Can you work these out from the model? Positions are in its coordinate system, mm. Face numbers are marked on the shaded views. A direction names the side the tool comes from. Give positions to 0.01 mm unless a question says otherwise; leave off trailing zeros. Loops run counter-clockwise (first coordinate to the right, second up) from the corner with the lowest first, then second, coordinate; pieces in that order, holes last. Notation, with made-up numbers: M -11.5,67 L -5.5,67 A23 ccw -5.5,90 Z; hole C 86,-6 d10. An arc over 180 degrees is marked long. Put each result on its own line as item: value. Start each with the question number.
1) Imagine slicing it at D-D (x = 5.5). Write out the boundary of the cut face in (y, z).
2) Imagine slicing it at B-B (z = 3.3). Write out the boundary of the cut face in (x, y).
3) For P1, Ø1.8, axis at x = 16.35, y = 10, coming from the -Z side; P2, Ø2, axis at x = 6, z = 0.5, coming from the -Y side; P3, Ø2, axis at y = 12, z = 1.5, coming from the -X side, each with a flat end and sliding along its axis, tell me the tip position at first contact or that it passes through.
4) Please list where these lines run through material, in increasing order: line 1 along Y through (x, z) = (26.35, 2.7); line 2 along X through (y, z) = (3, 0.8); line 3 along Y through (x, z) = (5, 3.45). Write a range as from..to.
5) Imagine slicing it at A-A (x = 26.35). Write out the boundary of the cut face in (y, z).
6) Imagine slicing it at C-C (y = 2.5). Write out the boundary of the cut face in (x, z), then the cut area to 3 significant figures.
7) For the marked faces 1, 2 and 3, which set-ups out of +Z, -Z, +X, -X, +Y, -Y let a thin tool reach every point of the face, with its end or its side?
8) If we mould it in two halves opening along Y, with no side actions, what happens to the marked faces 4, 5 and 6? For each: +Y half, -Y half, draft (parallel to the pull), parting line (faces both ways), or undercut.
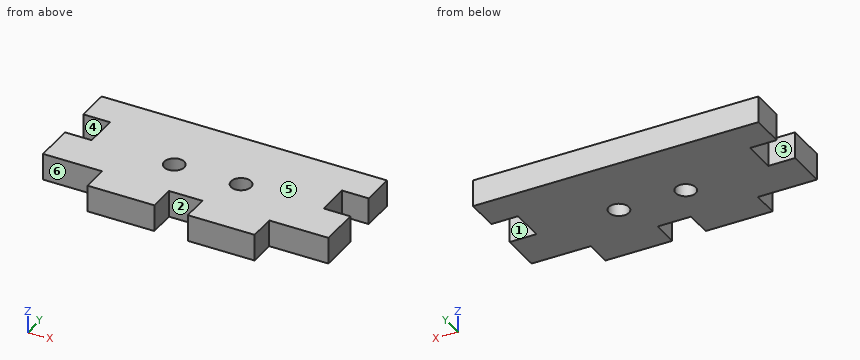
from build123d import *

# Parameters (mm, degrees)
SKETCH_1_W          = 42.7
SKETCH_1_H          = 20
EXTRUDE_1_DEPTH     = 4
SKETCH_2_R          = 1.5
SKETCH_2_W          = 8.85
SKETCH_2_H          = 4
SKETCH_2_W_2        = 5
SKETCH_2_W_3        = 4
SKETCH_2_H_2        = 5
CUT_EXTRUDE_1_DEPTH = 4


with BuildPart() as part:
    # Эскиз1 → Бобышка-Вытянуть1 (new body)
    with BuildSketch(Plane.XY):
        with Locations((21.35, 10)):
            Rectangle(SKETCH_1_W, SKETCH_1_H)
    extrude(amount=EXTRUDE_1_DEPTH)

    # Эскиз2 → Вырез-Вытянуть1 (cut)
    with BuildSketch(Plane.XY.offset(4)):
        with Locations((16.35, 10)):
            Circle(SKETCH_2_R)
        with Locations(Location((26.35, 10, 0), (0, 0, 180))):
            Circle(SKETCH_2_R)
        with Locations((4.425, 2)):
            Rectangle(SKETCH_2_W, SKETCH_2_H)
        with Locations((21.35, 2)):
            Rectangle(SKETCH_2_W_2, SKETCH_2_H)
        with Locations((38.275, 2)):
            Rectangle(SKETCH_2_W, SKETCH_2_H)
        with Locations((2, 12.5)):
            Rectangle(SKETCH_2_W_3, SKETCH_2_H_2)
        with Locations((40.7, 12.5)):
            Rectangle(SKETCH_2_W_3, SKETCH_2_H_2)
    extrude(amount=-CUT_EXTRUDE_1_DEPTH, mode=Mode.SUBTRACT)


solid = part.part
Recorded:
1. outline: M 4,0 L 20,0 L 20,4 L 4,4 Z
2. outline: M 0,4 L 8.85,4 L 8.85,0 L 18.85,0 L 18.85,4 L 23.85,4 L 23.85,0 L 33.85,0 L 33.85,4 L 42.7,4 L 42.7,10 L 38.7,10 L 38.7,15 L 42.7,15 L 42.7,20 L 0,20 L 0,15 L 4,15 L 4,10 L 0,10 Z; hole C 16.35,10 d3; hole C 26.35,10 d3
3. P1: through
3. P2: y = 4
3. P3: x = 4
4. line 1: 0..8.5, 11.5..20
4. line 2: 8.85..18.85, 23.85..33.85
4. line 3: 4..20
5. outline: M 0,0 L 8.5,0 L 8.5,4 L 0,4 Z; M 11.5,0 L 20,0 L 20,4 L 11.5,4 Z
6. outline: M 8.85,0 L 18.85,0 L 18.85,4 L 8.85,4 Z; M 23.85,0 L 33.85,0 L 33.85,4 L 23.85,4 Z
6. area: 80.0 mm²
7. face 1: +Z, -Z, +X
7. face 2: +Z, -Z, -Y
7. face 3: +Z, -Z, -X
8. face 4: undercut
8. face 5: draft
8. face 6: -Y half
